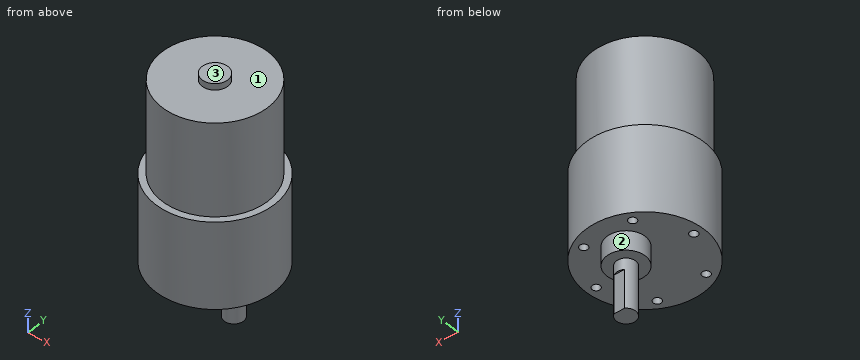
```python
from build123d import *

# Parameters (mm, degrees)
SKETCH1_R               = 18.5
BOSS_EXTRUDE1_DEPTH     = 27
SKETCH2_R               = 16.5
BOSS_EXTRUDE2_DEPTH     = 29
SKETCH3_R               = 4
BOSS_EXTRUDE3_DEPTH     = 2
M3_TAPPED_HOLE1_D       = 2.5
M3_TAPPED_HOLE1_DEPTH   = 8.5
M3_TAPPED_HOLE1_TIP     = 0.751075774
SKETCH4_R               = 6
BOSS_EXTRUDE4_DEPTH     = 6
SKETCH7_R               = 3
BOSS_EXTRUDE5_DEPTH     = 15.5
CUT_EXTRUDE1_DEPTH      = 1
CUT_EXTRUDE1_DEPTH_BACK = 12


with BuildPart() as part:
    # Sketch1 → Boss-Extrude1 (new body)
    with BuildSketch(Plane.XY):
        Circle(SKETCH1_R)
    extrude(amount=BOSS_EXTRUDE1_DEPTH)

    # Sketch2 → Boss-Extrude2 (add)
    with BuildSketch(Plane.XY.offset(27)):
        Circle(SKETCH2_R)
    extrude(amount=BOSS_EXTRUDE2_DEPTH)

    # Sketch3 → Boss-Extrude3 (add)
    with BuildSketch(Plane.XY.offset(56)):
        Circle(SKETCH3_R)
    extrude(amount=BOSS_EXTRUDE3_DEPTH)

    # M3 Tapped Hole1
    with Locations(Plane(origin=(15.5, -0.178765265, 0), x_dir=(-1, 0, 0), z_dir=(0, 0, -1))):
        with Locations((0, 0), (7.59518474, 13.512776391), (23.09518474, 13.691541656), (31, 0.35753053), (23.40481526, -13.155245861), (7.90481526, -13.334011126)):
            Hole(M3_TAPPED_HOLE1_D / 2, depth=M3_TAPPED_HOLE1_DEPTH)
            with Locations((0, 0, -(M3_TAPPED_HOLE1_DEPTH + M3_TAPPED_HOLE1_TIP / 2))):  # 118° drill point
                Cone(0, M3_TAPPED_HOLE1_D / 2, M3_TAPPED_HOLE1_TIP, mode=Mode.SUBTRACT)

    # Sketch4 → Boss-Extrude4 (add)
    with BuildSketch(Plane(origin=(0, 0, 0), x_dir=(-1, 0, 0), z_dir=(0, 0, -1))):
        with Locations((0, 7.000465539)):
            Circle(SKETCH4_R)
    extrude(amount=BOSS_EXTRUDE4_DEPTH)

    # Sketch7 → Boss-Extrude5 (add)
    with BuildSketch(Plane(origin=(0, 0, -6), x_dir=(-1, 0, 0), z_dir=(0, 0, -1))):
        with Locations((0, 7.000465539)):
            Circle(SKETCH7_R)
    extrude(amount=BOSS_EXTRUDE5_DEPTH)

    # Sketch8 → Cut-Extrude1 (cut, two sides)
    with BuildSketch(Plane(origin=(0, 0, -21.5), x_dir=(-1, 0, 0), z_dir=(0, 0, -1))) as cut_extrude1_sk:
        Polygon((-80.662185592, 9.500465539), (-1.658312395, 9.500465539), (1.658312395, 9.500465539), (80.662185592, 9.500465539), (80.662185592, 167.508211933), (-80.662185592, 167.508211933), align=None)
    extrude(amount=CUT_EXTRUDE1_DEPTH, mode=Mode.SUBTRACT)
    extrude(cut_extrude1_sk.sketch, amount=-CUT_EXTRUDE1_DEPTH_BACK, mode=Mode.SUBTRACT)


solid = part.part
```
Source: CAD feature listing. Evaluate the final solid. Frame: model axes, mm. Face numbers are marked on the shaded views. A direction names the side the tool comes from. Round coordinates to 2 decimals unless told otherwise and drop trailing zeros. Order: outer loops, then holes, each group sorted by start corner. A loop starts at its lowest first (then second) coordinate and runs counter-clockwise, first axis right, second up. Notation, with made-up numbers: (20, 18.5) -> (37, 18.5) arc R19 cw to (37, 30.5) -> close; hole circle Ø11 at (58, -27.5). An arc over 180 degrees is marked (long way). Use CSV: the item, a comma, the result in double quotes.
(1) Section D-D on x = -13. Return the cut outline in (y, z), and give its area (3 significant figures).
Report:
outline,"(-13.16, 0) -> (13.16, 0) -> (13.16, 27) -> (10.16, 27) -> (10.16, 56) -> (-10.16, 56) -> (-10.16, 27) -> (-13.16, 27) -> close"
area,"1,300 mm^2"
(2) Section B-B on z = -15.5. Return the cut outline in (x, y).
Report:
outline,"(-1.66, 9.5) arc R3 ccw (long way) to (1.66, 9.5) -> close"
(3) Section A-A on x = -0.5. Return the cut outline in (y, z).
Report:
outline,"(-18.49, 0) -> (1.02, 0) -> (1.02, -6) -> (4.04, -6) -> (4.04, -21.5) -> (9.5, -21.5) -> (9.5, -9.5) -> (9.96, -9.5) -> (9.96, -6) -> (12.98, -6) -> (12.98, 0) -> (18.49, 0) -> (18.49, 27) -> (16.49, 27) -> (16.49, 56) -> (3.97, 56) -> (3.97, 58) -> (-3.97, 58) -> (-3.97, 56) -> (-16.49, 56) -> (-16.49, 27) -> (-18.49, 27) -> close"
(4) Access query for the marked faces 1, 2 and 3. Directions: +Z, -Z, +X, -X, +Y, -Y. A direction counts if a zero-diameter tool reaches every point of the face in a straight line with its end or side. Return the directions, or none.
Report:
face 1,"+Z"
face 2,"-Z"
face 3,"+Z, +X, -X, +Y, -Y"
(5) Ray query, L1, parallel to Z at x = 12, y = 3; L2, parallel to Y at x = -14, z = 12; L3, parallel to Z at x = 5, y = 8. Return the intervals inside material, ascending.
Report:
L1,"0 to 56"
L2,"-12.09 to 12.09"
L3,"-6 to 56"
(6) Section C-C on z = 22. Return the cut outline in (x, y), and give its area (3 significant figures).
Report:
outline,"circle Ø37 at (0, 0)"
area,"1,080 mm^2"
(7) First-contact query: pin 1 Ø1 at (x, z) = (11, 19.5) entering from -Y; pin 2 Ø1.5 at (x, y) = (-15.5, 0.18) entering from -Z; pin 3 Ø6 at (y, z) = (9.5, 14.5) entering from +X. Flat tips, straight axial feed; report the tip coordinate or a pass-through.
Report:
pin 1,"y = -15.23"
pin 2,"z = 8.8"
pin 3,"x = 17.32"
